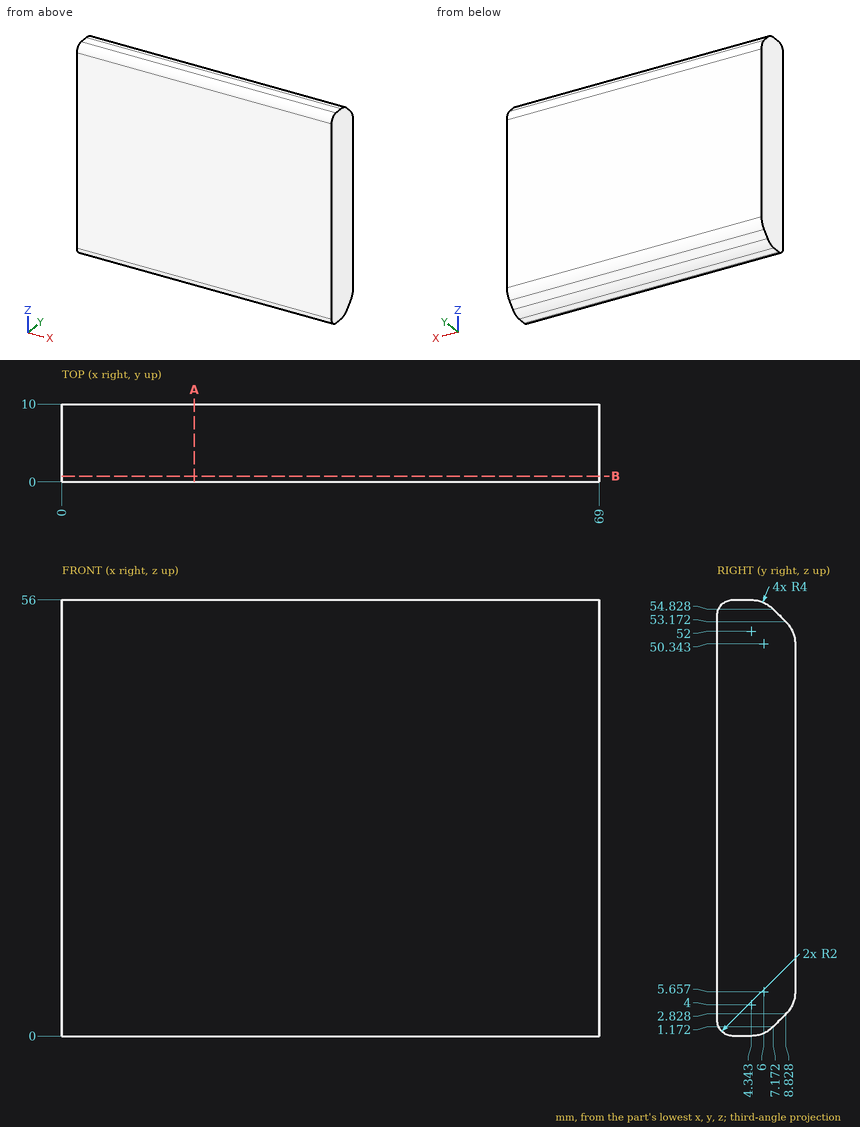
Print and shaded views of the part. All mm, measured from the part's lowest x, y and z. Give positions to 0.01 mm unless a question says otherwise; leave off trailing zeros. Loops run counter-clockwise (first coordinate to the right, second up) from the corner with the lowest first, then second, coordinate; pieces in that order, holes last. Notation, with made-up numbers: (-8, 11.5) -> (5, 11.5) arc R27 cw to (5, 34.5) -> close; hole circle Ø7 at (74.5, 68). An arc over 180 degrees is marked (long way). One line per question, with ' | ' between items. Start each with the question number.
1) Cut at A-A (x = 17). Give the cut face in (y, z), plus the area to 3 significant figures.
2) Cut at B-B (y = 0.75). Give the cut face in (x, z).
3) Probe L1, parallel to Z at x = 49.5, y = 9.25 (1 decimal); L2, parallel to Z at x = 12, y = 7.75. List the from-to ranges inside material, lowest first.
4) Pin check, flat tip, straight feed: pin 1 (4 mm diameter, centred on x = 46.5, y = 8, fed in from +Z). Stop position of the tip, or through.
Return value:
1) outline: (0, 2) arc R2 ccw to (2, 0) -> (4.34, 0) arc R4 ccw to (7.17, 1.17) -> (8.83, 2.83) arc R4 ccw to (10, 5.66) -> (10, 50.34) arc R4 ccw to (8.83, 53.17) -> (7.17, 54.83) arc R4 ccw to (4.34, 56) -> (2, 56) arc R2 ccw to (0, 54) -> close | area: 541 mm^2
2) outline: (0, 0.44) -> (69, 0.44) -> (69, 55.56) -> (0, 55.56) -> close
3) L1: 3.3 to 52.7 | L2: 1.75 to 54.25
4) pin 1: z = 55.64
